```python
from build123d import *

# Parameters (mm, degrees)
F0_R     = 9
F1_DEPTH = 3.6
F2_R     = 8
F3_DEPTH = 3
F4_R     = 9
F4_R_2   = 4.9
F5_DEPTH = 1.5


with BuildPart() as f1:
    # F0 (on Top) → F1 (new body)
    with BuildSketch(Plane.XY):
        Circle(F0_R)
    extrude(amount=F1_DEPTH)

    # F2 (on face) → F3 (cut)
    with BuildSketch(Plane.XY.offset(3.6)):
        Circle(F2_R)
    extrude(amount=-F3_DEPTH, mode=Mode.SUBTRACT)

    # F4 (on face) → F5 (join)
    with BuildSketch(Plane.XY.offset(3.6)):
        Circle(F4_R)
        Circle(F4_R_2, mode=Mode.SUBTRACT)
    extrude(amount=F5_DEPTH)


solid = f1.part
```
Could you check a few things on this model? Use its own coordinates, in mm. A direction names the side the tool comes from. Coordinates: 2 decimals unless noted, no trailing zeros. Loops run counter-clockwise (first coordinate to the right, second up) from the corner with the lowest first, then second, coordinate; pieces in that order, holes last.
1) Imagine slicing it at B-B (x = 7). List the corners of the cut face in (y, z) for me.
Reported:
outline: (-5.66, 0) - (5.66, 0) - (5.66, 5.1) - (-5.66, 5.1) - close; hole (-3.87, 0.6) - (3.87, 0.6) - (3.87, 3.6) - (-3.87, 3.6) - close
2) Imagine slicing it at C-C (y = 0). List the corners of the cut face in (x, z) for me, and give its area (3 significant figures).
Reported:
outline: (-9, 0) - (9, 0) - (9, 5.1) - (4.9, 5.1) - (4.9, 3.6) - (8, 3.6) - (8, 0.6) - (-8, 0.6) - (-8, 3.6) - (-4.9, 3.6) - (-4.9, 5.1) - (-9, 5.1) - close
area: 29.1 mm2
3) Please list where these lines run through material, in increasing order: line 1 along Z through (x, y) = (3, -6.5); line 2 along Y through (x, z) = (0, 1.7); line 3 along Y through (x, z) = (0, 4.5).
Reported:
line 1: z = 0 to 0.6, 3.6 to 5.1
line 2: y = -9 to -8, 8 to 9
line 3: y = -9 to -4.9, 4.9 to 9
4) Thinking about a two-plate mould opening in Z: for faces 3 (the face through (-1.062, -4.783, 4.34)), 4 (the face through (4, -4, 5.1)), 5 (the face through (0, 0, 0.6)), which applies, released by +Z, released by -Z, zero draft, split by the parting line, or undercut?
Reported:
face 3: zero draft
face 4: released by +Z
face 5: undercut
5) Will these pins go through, and if not, where does the flat tip stop? pin 1 Ø1.5 at (y, z) = (-5.5, 3.5) entering from +X; pin 2 Ø6 at (x, y) = (0, 0) entering from +Z; pin 3 Ø3 at (y, z) = (-4, 1.5) entering from +X.
Reported:
pin 1: stops at x = 7.64
pin 2: stops at z = 0.6
pin 3: stops at x = 8.65
6) Which directions (+Z, -Z, +X, -X, +Y, -Y) give clear straight access to the entire face, cutting with the end or side of a thin tool? Please do faces 1 (the face through (-1.172, 8.923, 2.514)), 2 (the face through (-0.1, -5.2, 3.6)).
Reported:
face 1: +Z, -Z
face 2: none
7) Imagine slicing it at A-A (z = 4.7). List the corners of the cut face in (x, y) for me, and give its area (3 significant figures).
Reported:
outline: circle Ø18 at (0, 0); hole circle Ø9.8 at (0, 0)
area: 179 mm2
